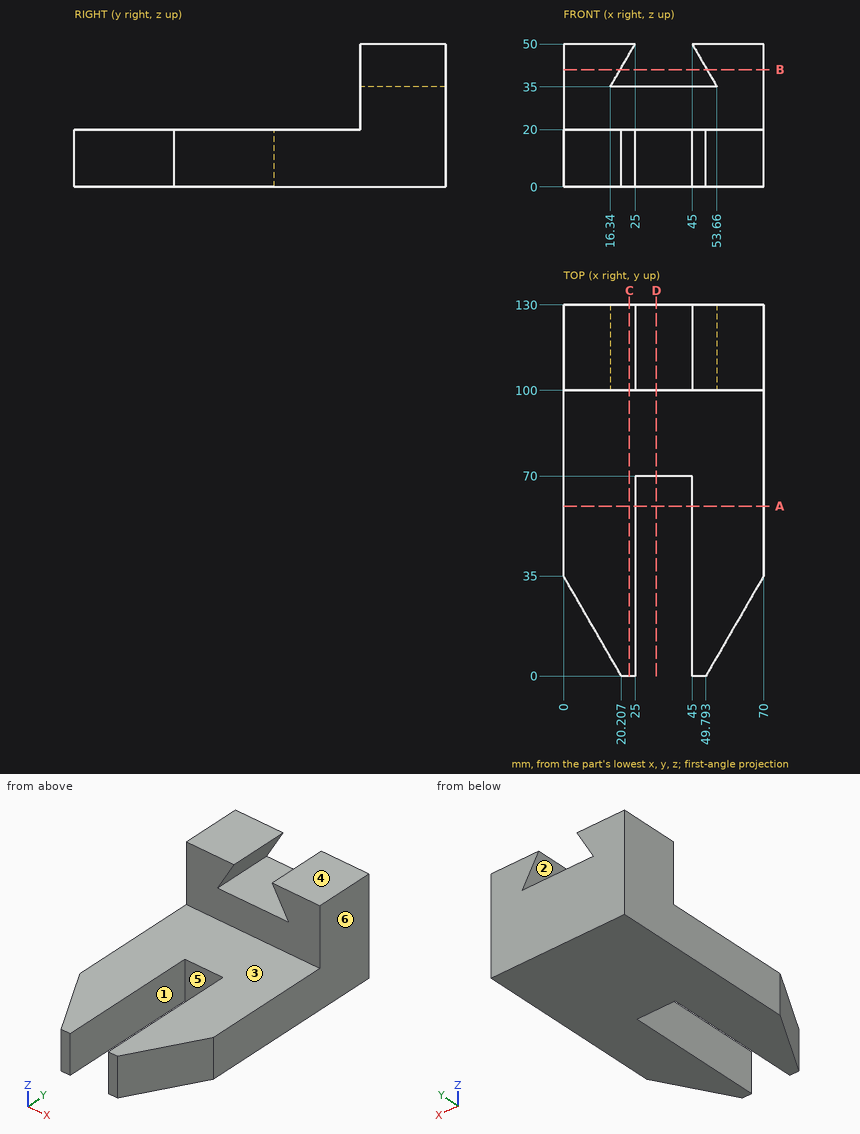
The drawing under review shows one solid part. Ordinate dimensions are in mm from its lowest x, y, z. A direction names the side the tool comes from. Give positions to 0.01 mm unless a question says otherwise; leave off trailing zeros. Loops run counter-clockwise (first coordinate to the right, second up) from the corner with the lowest first, then second, coordinate; pieces in that order, holes last. Notation, with made-up numbers: M 50.25,-3.5 L 79.25,-3.5 A13 ccw 79.25,0.5 Z; hole C 37.5,-36.5 d5. An arc over 180 degrees is marked long. One line per item, written item: value. Start each with the question number.
Q1. Draft analysis for pull direction X (two halves, no side actions). For the marked faces 4, 5 and 6, state which applies: released by +X, released by -X, zero draft, split by the parting line, or undercut.
Q2. Add section C-C (x = 23). Give the boundary of the cut face in (y, z).
Q3. Clearance check with flat-ended pins moving along their axes: pin 1 Ø10 at (x, z) = (15, 29.5) entering from -Y; pin 2 Ø10 at (x, y) = (11.5, 47.5) entering from +Z. State where each tip first meets the part, or that it passes through.
Q4. Add section D-D (x = 32.5). Give the boundary of the cut face in (y, z), and give its area (3 significant figures).
Q5. Add section B-B (z = 41). Give the boundary of the cut face in (x, y).
Q6. Add section A-A (y = 59.5). Give the boundary of the cut face in (x, z).
Q7. Machinability: for the marked faces 1, 2 and 3, which of the approach directions +Z, -Z, +X, -X, +Y, -Y give a long, thin tool a straight path to every point of the face, cutting with its end or side? Answer none if there is none.
Q8. For L1, parallel to Z at x = 10, y = 70.5; L2, parallel to X at y = 68.5, z = 4; L3, parallel to Y at x = 54.5, z = 23, list the stretches that pass through material, from the lowest coordinate up.
Reply:
1. face 4: zero draft
1. face 5: undercut
1. face 6: released by +X
2. outline: M 0,0 L 130,0 L 130,35 L 100,35 L 100,20 L 0,20 Z; M 100,46.54 L 130,46.54 L 130,50 L 100,50 Z
3. pin 1: y = 100
3. pin 2: z = 20
4. outline: M 70,0 L 130,0 L 130,35 L 100,35 L 100,20 L 70,20 Z
4. area: 1,650 mm²
5. outline: M 0,100 L 19.8,100 L 19.8,130 L 0,130 Z; M 50.2,100 L 70,100 L 70,130 L 50.2,130 Z
6. outline: M 0,0 L 25,0 L 25,20 L 0,20 Z; M 45,0 L 70,0 L 70,20 L 45,20 Z
7. face 1: +Z, -Z, -Y
7. face 2: +Y, -Y
7. face 3: +Z, +X, -X, -Y
8. L1: 0 to 20
8. L2: 0 to 25, 45 to 70
8. L3: 100 to 130
